For this review, take the finished solid that the model builds, in its own axes (mm). A direction names the side the tool comes from. Round coordinates to 2 decimals unless told otherwise and drop trailing zeros. Write each loop counter-clockwise with the first axis right and the second up, starting at its lowest first coordinate (ties: lowest second). Pieces come first, ordered by that corner, then holes. Notation, with made-up numbers: (4, -23) - (34, -23) arc R36 cw to (34, 12) - close; hole circle Ø11 at (17, 52). An arc over 180 degrees is marked (long way). Answer in a Markdown table with one row per item. Add a question column.
from build123d import *

# Parameters (mm, degrees)
SKETCH1_W           = 80
SKETCH1_H           = 96
BOSS_EXTRUDE1_DEPTH = 1.6
SKETCH3_W           = 25
SKETCH3_H           = 6.6
BOSS_EXTRUDE2_DEPTH = 5


with BuildPart() as part:
    # Sketch1 → Boss-Extrude1 (new body)
    with BuildSketch(Plane.XY.offset(-42.6)):
        Rectangle(SKETCH1_W, SKETCH1_H)
    extrude(amount=BOSS_EXTRUDE1_DEPTH)

    # Sketch3 → Boss-Extrude2 (add)
    with BuildSketch(Plane.XY.offset(-42.6)):
        with Locations((0, 39.3)):
            Rectangle(SKETCH3_W, SKETCH3_H)
        with Locations((0, 27.3)):
            Rectangle(SKETCH3_W, SKETCH3_H)
        with Locations((0, 15.3)):
            Rectangle(SKETCH3_W, SKETCH3_H)
        with Locations((0, 3.3)):
            Rectangle(SKETCH3_W, SKETCH3_H)
        with Locations((0, -8.7)):
            Rectangle(SKETCH3_W, SKETCH3_H)
        with Locations((0, -20.7)):
            Rectangle(SKETCH3_W, SKETCH3_H)
        with Locations((0, -32.7)):
            Rectangle(SKETCH3_W, SKETCH3_H)
    extrude(amount=BOSS_EXTRUDE2_DEPTH)


solid = part.part
Q1. Add section C-C on y = -7. State the section outline as (x, z) points, then the cut area to 3 significant figures.
Q2. Tool access review of faces 1 (the face through (-12.5, -9, -39)), 2 (the face through (0, -24, -39)), 3 (the face through (12.5, -21, -39)), 4 (the face through (0, 3, -37.6)): name each direction out of +Z, -Z, +X, -X, +Y, -Y from which nothing blocks a thin tool from reaching the whole face with its end or side.
Q3. Add section D-D on x = -32. State the section outline as (y, z) points.
Q4. To check wall thickness, follow probe 1 along X at (y, z) = (-10, -40.9); probe 2 along Z at (x, y) = (36, 26). State the ranges of each line that lie inside material, in increasing order.
Q5. Insertion check: pin 1 Ø2.5 at (y, z) = (16.5, -39) entering from -X; pin 2 Ø1.7 at (x, z) = (1, -40) entering from -Y; pin 3 Ø1 at (x, y) = (29, 31) entering from +Z. Each pin has a flat end and moves straight along its axis. Give the tip position at first contact, or say it passes through.
Q6. Draft analysis for pull direction Y (two halves, no side actions). For faces 5 (the face through (0, -36, -39)), 6 (the face through (0, -12, -39)), 7 (the face through (0, -21, -37.6)), state which applies: released by +Y, released by -Y, zero draft, split by the parting line, or undercut.
Q7. Add section A-A on z = -39.1. State the section outline as (x, y) points.
Answer sheet:
| question | item | result |
|---|---|---|
| 1 | outline | (-40, -42.6) - (40, -42.6) - (40, -41) - (12.5, -41) - (12.5, -37.6) - (-12.5, -37.6) - (-12.5, -41) - (-40, -41) - close |
| 1 | area | 213 mm² |
| 2 | face 1 | +Z, -X, +Y, -Y |
| 2 | face 2 | +Z, +X, -X |
| 2 | face 3 | +Z, +X, +Y, -Y |
| 2 | face 4 | +Z, +X, -X, +Y, -Y |
| 3 | outline | (-48, -42.6) - (48, -42.6) - (48, -41) - (-48, -41) - close |
| 4 | probe 1 | x = -12.5 to 12.5 |
| 4 | probe 2 | z = -42.6 to -41 |
| 5 | pin 1 | stops at x = -12.5 |
| 5 | pin 2 | stops at y = -36 |
| 5 | pin 3 | stops at z = -41 |
| 6 | face 5 | released by -Y |
| 6 | face 6 | undercut |
| 6 | face 7 | zero draft |
| 7 | outline | (-12.5, -36) - (12.5, -36) - (12.5, -29.4) - (-12.5, -29.4) - close; (-12.5, -24) - (12.5, -24) - (12.5, -17.4) - (-12.5, -17.4) - close; (-12.5, -12) - (12.5, -12) - (12.5, -5.4) - (-12.5, -5.4) - close; (-12.5, 0) - (12.5, 0) - (12.5, 6.6) - (-12.5, 6.6) - close; (-12.5, 12) - (12.5, 12) - (12.5, 18.6) - (-12.5, 18.6) - close; (-12.5, 24) - (12.5, 24) - (12.5, 30.6) - (-12.5, 30.6) - close; (-12.5, 36) - (12.5, 36) - (12.5, 42.6) - (-12.5, 42.6) - close |
